Read the model definition and answer for the solid it produces. Units are mm, in the model's axes. A direction names the side the tool comes from. Give positions to 0.01 mm unless a question says otherwise; leave off trailing zeros. Order: outer loops, then holes, each group sorted by start corner. A loop starts at its lowest first (then second) coordinate and runs counter-clockwise, first axis right, second up. Notation, with made-up numbers: (74, 47.5) -> (112, 47.5) arc R26 ccw to (112, 61.5) -> close; hole circle Ø5 at (-19, 28.25). An arc over 180 degrees is marked (long way). Answer as CSV lines item,"result". Start each with the question number.
1) Find section A-A (x = -3). Determine the outline of the cut face in (y, z), and give its area (3 significant figures).
2) Straight lines are drawn through the part: L1, parallel to Z at x = 28.25, y = 0; L2, parallel to Y at x = 42.25, z = 0; L3, parallel to Y at x = 34.25, z = 0. For each, find the intervals that lie inside material, in ascending order. Write a range as from..to.
3) Flat-ended cylindrical pins translate along their axes: pin 1 Ø3 at (x, z) = (-9, 5) entering from +Y; pin 2 Ø5 at (x, z) = (19.5, 4.5) entering from +Y; pin 3 Ø1 at (x, y) = (-8, -6.5) entering from +Z. Find the tip coordinate at first contact, or state that the pin passes through.
4) For faces 4 (the face through (35.592, -6.466, -2.681)), 5 (the face through (-42.198, 0, 0)), determine the directions among +Z, -Z, +X, -X, +Y, -Y from which every point of the face is accessible in a straight line to the end or side of a thin tool.
5) The mould has two halves that part along Y. Classify faces 1 (the face through (17.33, -0.26, -1.19)), 2 (the face through (50.802, 5.2, -5.2)), 3 (the face through (-8.181, -0.66, -14.985)): +Y half, -Y half, draft (parallel to the pull), parting line (faces both ways), or undercut.
```python
from build123d import *

# Parameters (mm, degrees)
F2_R     = 7
F3_DEPTH = 30
F5_D     = 14
F5_DEPTH = 30
F5_TIP   = 4.2060243332


with BuildPart() as f1:
    # F0 (on Front) → F1 (revolve)
    with BuildSketch(Plane.XZ):
        Polygon((-42.1976023009, 15), (-42.1976023009, 0), (-20.7868143916, 0), (26.8023976991, 0), (26.8023976991, 15), align=None)
        Polygon((26.8023976991, 15), (26.8023976991, 0), (50.8023976991, 0), (50.8023976991, 12), align=None)
    revolve(axis=Axis((4.7784452844, 0, 0), (1, 0, 0)))

    # F2 (on face) → F3 (join)
    with BuildSketch(Plane.YZ.offset(50.8023976991)):
        Circle(F2_R)
    extrude(amount=-F3_DEPTH)

    # F5
    with Locations(Plane.YZ.offset(50.8023976991)):
        with Locations((0, 0)):
            Hole(F5_D / 2, depth=F5_DEPTH)
            with Locations((0, 0, -(F5_DEPTH + F5_TIP / 2))):  # 118° drill point
                Cone(0, F5_D / 2, F5_TIP, mode=Mode.SUBTRACT)


solid = f1.part
```
Findings below:
1,outline,"circle Ø30 at (0, 0)"
1,area,"707 mm²"
2,L1,"-14.82..-7, 7..14.82"
2,L2,"-13.07..-7, 7..13.07"
2,L3,"-14.07..-7, 7..14.07"
3,pin 1,"y = 14.59"
3,pin 2,"y = 14.87"
3,pin 3,"z = 13.75"
4,face 4,"+X"
4,face 5,"+Z, -Z, -X, +Y, -Y"
5,face 1,"undercut"
5,face 2,"draft"
5,face 3,"parting line"
